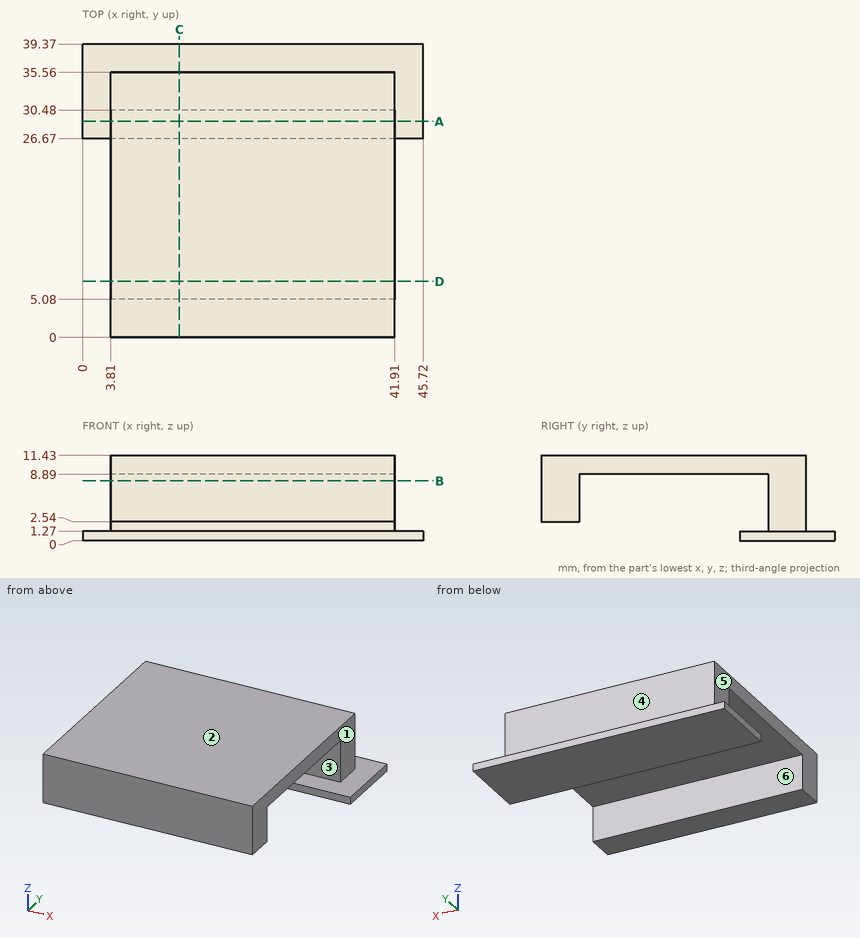
Geometry check sheet. Reference: drawing and pictorial views, mm from the part's lowest x, y, z. A direction names the side the tool comes from. Give positions to 0.01 mm unless a question says otherwise; leave off trailing zeros. Order: outer loops, then holes, each group sorted by start corner. A loop starts at its lowest first (then second) coordinate and runs counter-clockwise, first axis right, second up. Notation, with made-up numbers: (44, -13) - (98, -13) arc R29 cw to (98, 20) - close; hole circle Ø7 at (-14.75, -19). An arc over 180 degrees is marked (long way). Answer as CSV lines item,"result". Start each with the question number.
Item 1: Access from +Z, -Z, +X, -X, +Y, -Y to the whole of each face (thin tool, end or side, straight path). Record for the marked faces 4, 5 and 6.
Item 2: Section check D-D, the plane y = 7.5. Record the boundary of the cut face in (x, z).
Item 3: Section check A-A, the plane y = 29. Record the boundary of the cut face in (x, z), plus the area to 3 significant figures.
Item 4: Section check C-C, the plane x = 13. Record the boundary of the cut face in (y, z).
Item 5: Section check B-B, the plane z = 8. Record the boundary of the cut face in (x, y), plus the area to 3 significant figures.
Item 6: Mould release check, pull along Z, two halves, no side actions. Record for the marked faces 1, 2 and 3: released by +Z, released by -Z, zero draft, split by the parting line, or undercut.
Item 7: Gauge pin test, flat ends, axial feed: pin 1 (4 mm diameter, centred on x = 41, z = 5, fed in from +Y); pin 2 (4 mm diameter, centred on x = 17, y = 3.5, fed in from -Z); pin 3 (1.4 mm diameter, centred on x = 16.5, z = 1, fed in from -Y); pin 4 (2.5 mm diameter, centred on x = 26.5, z = 5.5, fed in from -Y). Record the tip position at first contact, or that the pin passes through.
Item 8: Material ranges on L1, parallel to Y at x = 20, z = 8.75; L2, parallel to Z at x = 26, y = 14; L3, parallel to Z at x = 23, y = 37, recorded low to high.
Filled in:
1,face 4,"+Z, +X, -X, +Y"
1,face 5,"+Z, -X, +Y, -Y"
1,face 6,"-Z, +X, -X"
2,outline,"(3.81, 8.89) - (41.91, 8.89) - (41.91, 11.43) - (3.81, 11.43) - close"
3,outline,"(0, 0) - (45.72, 0) - (45.72, 1.27) - (0, 1.27) - close; (3.81, 8.89) - (41.91, 8.89) - (41.91, 11.43) - (3.81, 11.43) - close"
3,area,"155 mm^2"
4,outline,"(0, 2.54) - (5.08, 2.54) - (5.08, 8.89) - (30.48, 8.89) - (30.48, 1.27) - (26.67, 1.27) - (26.67, 0) - (39.37, 0) - (39.37, 1.27) - (35.56, 1.27) - (35.56, 11.43) - (0, 11.43) - close"
5,outline,"(3.81, 0) - (41.91, 0) - (41.91, 5.08) - (3.81, 5.08) - close; (3.81, 30.48) - (41.91, 30.48) - (41.91, 35.56) - (3.81, 35.56) - close"
5,area,"387 mm^2"
6,face 1,"zero draft"
6,face 2,"released by +Z"
6,face 3,"undercut"
7,pin 1,"y = 35.56"
7,pin 2,"z = 2.54"
7,pin 3,"y = 26.67"
7,pin 4,"y = 0"
8,L1,"0 to 5.08, 30.48 to 35.56"
8,L2,"8.89 to 11.43"
8,L3,"0 to 1.27"
